Design review of the part built by this model. Coordinates are the model's own, in mm. Face numbers are marked on the shaded views. A direction names the side the tool comes from. Give positions to 0.01 mm unless a question says otherwise; leave off trailing zeros. Write each loop counter-clockwise with the first axis right and the second up, starting at its lowest first coordinate (ties: lowest second). Pieces come first, ordered by that corner, then holes. Notation, with made-up numbers: M 84,17.5 L 129,17.5 A9 ccw 129,24.5 Z; hole C -20.75,4 d5. An arc over 180 degrees is marked long. Use one line per item in the form item = value. Start each with the question number.
from build123d import *

# Parameters (mm, degrees)
F0_W     = 40
F0_H     = 40
F1_DEPTH = 30
F2_W     = 20
F2_H     = 20
F2_W_2   = 16.331926
F2_H_2   = 16.661864
F2_H_3   = 15.507082
F2_W_3   = 16.661866
F3_DEPTH = 30
F4_R     = 5


with BuildPart() as f1:
    # F0 (on Front) → F1 (new body)
    with BuildSketch(Plane.XZ):
        Rectangle(F0_W, F0_H)
    extrude(amount=F1_DEPTH)

    # F2 (on face) → F3 (cut, through all)
    with BuildSketch(Plane.XZ.offset(30)):
        with Locations((10, 10)):
            Rectangle(F2_W, F2_H)
        with Locations((-10.085583, 10.036508)):
            Rectangle(F2_W_2, F2_H_2)
        with Locations((-10.085583, -10.00722)):
            Rectangle(F2_W_2, F2_H_3)
        with Locations((9.710691, -10.00722)):
            Rectangle(F2_W_3, F2_H_3)
    extrude(amount=-F3_DEPTH, mode=Mode.SUBTRACT)

    # F4
    f4_edges = [f1.edges().sort_by_distance(p)[0] for p in [
        (0, -15, 0),
        (-18.251546, -15, 18.36744),
        (-1.91962, -15, 18.36744),
        (-18.251546, -15, 1.705576),
        (-1.91962, -15, 1.705576),
        (-1.91962, -15, -17.760761),
        (18.041624, -15, -17.760761),
        (18.041624, -15, -2.253679),
        (-1.91962, -15, -2.253679),
        (-18.251546, -15, -2.253679),
        (1.379758, -15, -2.253679),
        (-18.251546, -15, -17.760761),
        (1.379758, -15, -17.760761),
    ]]
    fillet(f4_edges, radius=F4_R)


solid = f1.part
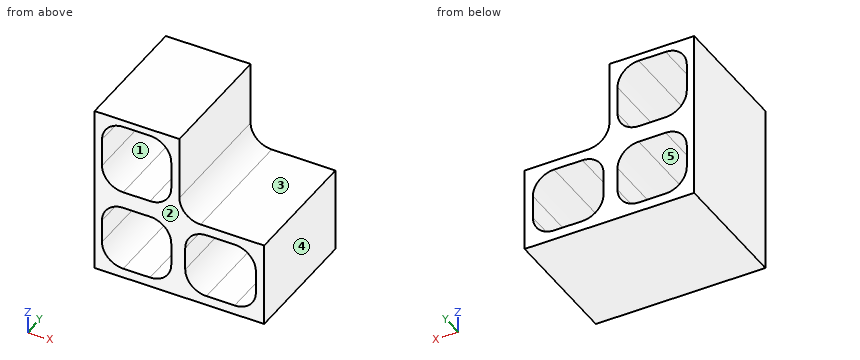
1. Clearance check with flat-ended pins moving along their axes: pin 1 Ø12 at (x, y) = (11, -18.5) entering from +Z; pin 2 Ø7.5 at (y, z) = (-21, 12.5) entering from +X. State where each tip first meets the part, or that it passes through.
2. We need section C-C (z = 12). State the section outline as (x, y) points, and give its area (3 significant figures).
3. Draft analysis for pull direction X (two halves, no side actions). For the marked faces 3, 4 and 5, state which applies: pulls with the +X half, pulls with the -X half, needs draft (parallel to the pull), parting line crosses it, or undercut.
4. For the marked faces 1 and 2, list the 3-axis set-ups (+Z, -Z, +X, -X, +Y, -Y) from which the entire face can be reached by the end or side of a thin tool; tool diameter is ignored.
5. To check wall thickness, follow L1, parallel to X at y = -3, z = -10; L2, parallel to Z at x = -13, y = -16; L3, parallel to X at y = -2.25, z = -13. State the ranges of each line that lie inside material, in increasing order.
6. We need section A-A (y = -16.5). Give the number of separate pieces and of enclosed holes in the cut face, and give its area (3 significant figures).
7. We need section D-D (x = 16). State the section outline as (y, z) points, and give its area (3 significant figures).
8. We need section B-B (x = -9). State the section outline as (y, z) points, and give its area (3 significant figures).
Answer block:
q1.pin_1 = 0
q1.pin_2 = 0
q2.outline = M -20,-30 L -18.25,-30 L -18.25,0 L -20,0 Z; M -1.92,-30 L 0,-30 L 0,0 L -1.92,0 Z
q2.area = 110 mm^2
q3.face_3 = needs draft
q3.face_4 = pulls with the +X half
q3.face_5 = undercut
q4.face_1 = +Y, -Y
q4.face_2 = +Z, -Z, +X, -X, -Y
q5.L1 = -20 to -18.25, -1.92 to 1.38, 18.04 to 20
q5.L2 = -20 to -17.76, -2.25 to 1.71, 18.37 to 20
q5.L3 = -20 to -18.25, -1.93 to 1.39, 18.04 to 20
q6.separate_pieces = 1
q6.enclosed_holes = 3
q6.area = 486 mm^2
q7.outline = M -30,-20 L 0,-20 L 0,-16.79 L -30,-16.79 Z; M -30,-3.22 L 0,-3.22 L 0,0 L -30,0 Z
q7.area = 193 mm^2
q8.outline = M -30,-20 L 0,-20 L 0,-17.76 L -30,-17.76 Z; M -30,-2.25 L 0,-2.25 L 0,1.71 L -30,1.71 Z; M -30,18.37 L 0,18.37 L 0,20 L -30,20 Z
q8.area = 235 mm^2
